```python
from build123d import *

# Parameters (mm, degrees)
SKETCH1_R               = 1.5
BOSS_EXTRUDE1_DEPTH     = 2
SKETCH2_W               = 7
SKETCH2_H               = 9
BOSS_EXTRUDE2_DEPTH     = 5
SKETCH2_3_W             = 1.9
SKETCH2_3_H             = 9
BOSS_EXTRUDE3_DEPTH     = 11
BOSS_EXTRUDE4_DEPTH     = 11
CUT_EXTRUDE1_DEPTH      = 17.718253497
CUT_EXTRUDE1_DEPTH_BACK = 17.718253497
SKETCH5_R               = 2.966905055
CUT_EXTRUDE2_DEPTH      = 11


with BuildPart() as part:
    # Sketch1 → Boss-Extrude1 (new body)
    with BuildSketch(Plane.XY):
        with BuildLine():
            Line((-5, 4.5), (5, 4.5))
            ThreePointArc((5, 4.5), (9.5, 0), (5, -4.5))
            Line((5, -4.5), (-5, -4.5))
            ThreePointArc((-5, -4.5), (-9.5, 0), (-5, 4.5))
        make_face()
        with Locations((-5, 0)):
            Circle(SKETCH1_R, mode=Mode.SUBTRACT)
        with Locations(Location((5, 0, 0), (0, 0, 180))):
            Circle(SKETCH1_R, mode=Mode.SUBTRACT)
    extrude(amount=BOSS_EXTRUDE1_DEPTH)

    # Sketch2 → Boss-Extrude2 (add)
    with BuildSketch(Plane.XY.offset(2)):
        Rectangle(SKETCH2_W, SKETCH2_H)
    extrude(amount=BOSS_EXTRUDE2_DEPTH)

    # Sketch2<3> → Boss-Extrude3 (add)
    with BuildSketch(Plane.XY.offset(2)):
        with Locations((-2.55, 0)):
            Rectangle(SKETCH2_3_W, SKETCH2_3_H)
        with Locations((2.55, 0)):
            Rectangle(SKETCH2_3_W, SKETCH2_3_H)
    extrude(amount=BOSS_EXTRUDE3_DEPTH)

    # Sketch3 → Boss-Extrude4 (add)
    with BuildSketch(Plane.XY.offset(2)):
        with BuildLine():
            Line((-3.5, 4.5), (-5, 4.5))
            ThreePointArc((-5, 4.5), (-6.85727317, 4.098845737), (-8.38341165, 2.966905055))
            Line((-8.38341165, 2.966905055), (-3.5, 2.966905055))
            Line((-3.5, 2.966905055), (-3.5, 4.5))
        make_face()
        with BuildLine():
            Line((-3.5, -2.966905055), (-8.38341165, -2.966905055))
            ThreePointArc((-8.38341165, -2.966905055), (-6.85727317, -4.098845737), (-5, -4.5))
            Line((-5, -4.5), (-3.5, -4.5))
            Line((-3.5, -4.5), (-3.5, -2.966905055))
        make_face()
        with BuildLine():
            Line((3.5, -4.5), (5, -4.5))
            ThreePointArc((5, -4.5), (6.85727317, -4.098845737), (8.38341165, -2.966905055))
            Line((8.38341165, -2.966905055), (3.5, -2.966905055))
            Line((3.5, -2.966905055), (3.5, -4.5))
        make_face()
        with BuildLine():
            Line((3.5, 2.966905055), (8.38341165, 2.966905055))
            ThreePointArc((8.38341165, 2.966905055), (6.85727317, 4.098845737), (5, 4.5))
            Line((5, 4.5), (3.5, 4.5))
            Line((3.5, 4.5), (3.5, 2.966905055))
        make_face()
    extrude(amount=BOSS_EXTRUDE4_DEPTH)

    # Sketch4 → Cut-Extrude1 (cut, two sides: drawn at the far end of the back side and taken through both)
    with BuildSketch(Plane(origin=(0, 0, 0), x_dir=(1, 0, 0), z_dir=(0, 1, 0)).offset(-CUT_EXTRUDE1_DEPTH_BACK)):
        with BuildLine():
            Line((-8.38341165, -2), (-12.296417953, -13.182835844))
            Line((-12.296417953, -13.182835844), (-6.078905494, -14.351094555))
            Line((-6.078905494, -14.351094555), (-5, -13))
            add(Edge.make_bspline(
                [(-8.38341165, -2), (-5.354296854, -5.236477868), (-5, -13)],
                knots=[0, 0, 0, 1, 1, 1], degree=2))
        make_face()
        with BuildLine():
            Line((5, -13), (8.38341165, -14.707512466))
            Line((8.38341165, -14.707512466), (10.514328395, -13.974875648))
            Line((10.514328395, -13.974875648), (8.38341165, -2))
            add(Edge.make_bspline(
                [(8.38341165, -2), (5.354296854, -5.236477868), (5, -13)],
                knots=[0, 0, 0, 1, 1, 1], degree=2))
        make_face()
    extrude(amount=CUT_EXTRUDE1_DEPTH + CUT_EXTRUDE1_DEPTH_BACK, mode=Mode.SUBTRACT)

    # Sketch5 → Cut-Extrude2 (cut)
    with BuildSketch(Plane.XY.offset(13)):
        with Locations((-5, 0)):
            Circle(SKETCH5_R)
        with Locations((5, 0)):
            Circle(SKETCH5_R)
    extrude(amount=-CUT_EXTRUDE2_DEPTH, mode=Mode.SUBTRACT)


solid = part.part
```
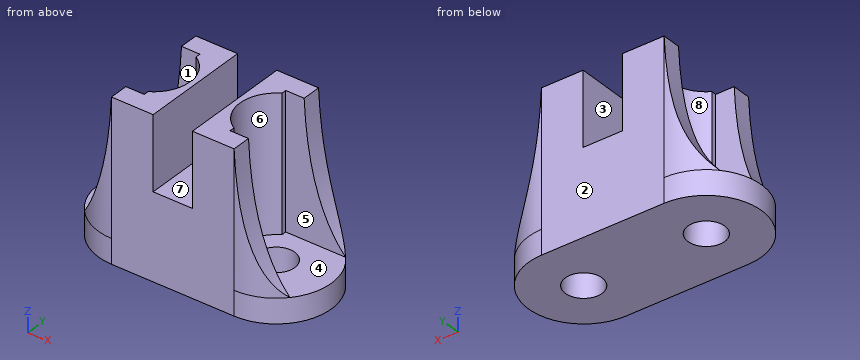
For this review, take the finished solid that the model builds, in its own axes (mm). Face numbers are marked on the shaded views. A direction names the side the tool comes from. Round coordinates to 2 decimals unless told otherwise and drop trailing zeros. Write each loop counter-clockwise with the first axis right and the second up, starting at its lowest first coordinate (ties: lowest second). Pieces come first, ordered by that corner, then holes. Notation, with made-up numbers: (49.25, -29) -> (75.25, -29) arc R29 cw to (75.25, 8) -> close; hole circle Ø9 at (37, -28). An arc over 180 degrees is marked (long way). Use one line per item in the form item = value.
Q1. Consider section A-A (y = 0). State the section outline as (x, z) points, then the cut area to 3 significant figures.
Resolved:
outline = (-9.5, 0) -> (-6.5, 0) -> (-6.5, 2) -> (-9.5, 2) -> close; (-3.5, 0) -> (3.5, 0) -> (3.5, 2) -> (2.03, 2) -> (2.03, 13) -> (1.6, 13) -> (1.6, 7) -> (-1.6, 7) -> (-1.6, 13) -> (-2.03, 13) -> (-2.03, 2) -> (-3.5, 2) -> close; (6.5, 0) -> (9.5, 0) -> (9.5, 2) -> (6.5, 2) -> close
area = 51.5 mm²
Q2. Consider section C-C (y = 2). State the section outline as (x, z) points.
Resolved:
outline = (-9.03, 0) -> (9.03, 0) -> (9.03, 2) -> (2.81, 2) -> (2.81, 13) -> (1.6, 13) -> (1.6, 7) -> (-1.6, 7) -> (-1.6, 13) -> (-2.81, 13) -> (-2.81, 2) -> (-9.03, 2) -> close
Q3. Machinability: for the marked faces 1, 2, 3 and 4, which of the approach directions +Z, -Z, +X, -X, +Y, -Y give a long, thin tool a straight path to every point of the face, cutting with its end or side? Answer none if there is none.
Resolved:
face_1 = +Z, -X
face_2 = +Z, -Z, +X, -X, +Y
face_3 = +Z, +Y, -Y
face_4 = +Z, +X
Q4. To check wall thickness, follow probe 1 along Y at (x, z) = (5, 1); probe 2 along Y at (x, z) = (-4.25, 8.5); probe 3 along X at (y, z) = (2.75, 4.25). State the ranges of each line that lie inside material, in increasing order. Write a range as from..to.
Resolved:
probe_1 = -4.5..-1.5, 1.5..4.5
probe_2 = -4.5..-2.97, 2.97..4.5
probe_3 = -3.5..3.5
Q5. Consider section D-D (y = -1.25). State the section outline as (x, z) points, then the cut area to 3 significant figures.
Resolved:
outline = (-9.32, 0) -> (-5.83, 0) -> (-5.83, 2) -> (-9.32, 2) -> close; (-4.17, 0) -> (4.17, 0) -> (4.17, 2) -> (2.31, 2) -> (2.31, 13) -> (1.6, 13) -> (1.6, 7) -> (-1.6, 7) -> (-1.6, 13) -> (-2.31, 13) -> (-2.31, 2) -> (-4.17, 2) -> close; (5.83, 0) -> (9.32, 0) -> (9.32, 2) -> (5.83, 2) -> close
area = 62.3 mm²
Q6. Clearance check with flat-ended pins moving along their axes: pin 1 Ø1 at (x, y) = (0, 3) entering from +Z; pin 2 Ø5 at (x, y) = (-5, 0) entering from +Z; pin 3 Ø2.5 at (x, z) = (7, 7) entering from -Y. State where each tip first meets the part, or that it passes through.
Resolved:
pin_1 = 7
pin_2 = 2
pin_3 = -4.44
Q7. The part is to be moulded in two halves that separate along X. For the marked faces 5, 6, 7 and 8, say which applies: released by +X, released by -X, zero draft, split by the parting line, or undercut.
Resolved:
face_5 = zero draft
face_6 = released by +X
face_7 = undercut
face_8 = released by -X
Q8. Consider section B-B (x = 2.5). State the section outline as (y, z) points, then the cut area to 3 significant figures.
Resolved:
outline = (-4.5, 0) -> (4.5, 0) -> (4.5, 13) -> (1.6, 13) -> (1.6, 2) -> (-1.6, 2) -> (-1.6, 13) -> (-4.5, 13) -> close
area = 81.9 mm²
